Source: CAD feature listing. Evaluate the final solid. Frame: model axes, mm. A direction names the side the tool comes from. Give positions to 0.01 mm unless a question says otherwise; leave off trailing zeros. Loops run counter-clockwise (first coordinate to the right, second up) from the corner with the lowest first, then second, coordinate; pieces in that order, holes last. Notation, with made-up numbers: (35.25, -24.5) -> (73.25, -24.5) arc R21 ccw to (73.25, -19.5) -> close; hole circle Ø7 at (-19.75, -4.75). An arc over 180 degrees is marked (long way). Return JSON: item names as keys, results as strings. Group by question number.
(1) Pin query (flat end, axial travel): pin 1 (5 mm diameter, centred on y = -482.5, z = 15.5, fed in from +X); pin 2 (1 mm diameter, centred on y = -469.5, z = 15.5, fed in from -X); pin 3 (8 mm diameter, centred on x = -2.5, z = 4, fed in from -Y); pin 4 (10 mm diameter, centred on x = -100.5, z = 16, fed in from -Y). Return the tip coordinate at first contact, or that it passes through.
(2) Cut plane B-B on y = -56.5. Return loops of the section in (x, z), then the cut area to 3 significant figures.
(3) Ray query, line 1 (Y direction, x = -10, z = 11); line 2 (X direction, y = -374.5, z = 24.25). Return the intervals inside material, ascending. Write a range as from..to.
(4) Cut plane A-A on x = -73. Return loops of the section in (y, z).
(5) Access query for faces 5 (the face through (-101.6, 661, 13)), 6 (the face through (-153, 317.5, 13)), 7 (the face through (127, -660, 13)). Directions: +Z, -Z, +X, -X, +Y, -Y. A direction counts if a zero-diameter tool reaches every point of the face in a straight line with its end or side. Return the directions, or none.
(6) Draft query along X for faces 1 (the face through (-152, -12.7, 13)), 2 (the face through (127, -455, 13)), 3 (the face through (-127, 455, 13)), 4 (the face through (1, -317.5, 13)). Return one class per face: released by +X, released by -X, zero draft, split by the parting line, or undercut.
(7) Cut plane C-C on z = 16.5. Give the number of separate pieces and of enclosed holes in the cut face, then the cut area to 3 significant figures.
Autodesk Inventor part; units mm, degrees
ref_plane "YZ Plane" through (0, 0, 0) normal (1, 0, 0) x (0, 1, 0)
ref_plane "XZ Plane" through (0, 0, 0) normal (0, 1, 0) x (-1, 0, 0)
ref_plane "XY Plane" through (0, 0, 0) normal (0, 0, 1) x (1, 0, 0)
sketch "Sketch1" plane through (0, 0, 0) normal (0, 0, 1) x (1, 0, 0)
  line L0 (-127, 698.5) -> (-101.6, 698.5)
  line L1 (-101.6, 698.5) -> (-101.6, -698.5)
  line L2 (-101.6, -698.5) -> (-127, -698.5)
  line L3 (-127, -698.5) -> (-127, 698.5)
  line L4 (101.6, 698.5) -> (127, 698.5)
  line L5 (127, 698.5) -> (127, -698.5)
  line L6 (127, -698.5) -> (101.6, -698.5)
  line L7 (101.6, -698.5) -> (101.6, 698.5)
  line L8 (0, 0) -> (0, 143.5331) construction
  line L9 (0, 0) -> (-211.7363, 0) construction
  dimension "d0" = 25.4
  dimension "d1" = 1397
  dimension "d2" = 203.2
extrude "Extrusion1" add sketch "Sketch1" along normal blind 25.4
sketch "Sketch2" plane through (0, 0, 25.4) normal (0, 0, 1) x (1, 0, 0)
  line L0 (-177.8, 622.3) -> (177.8, 622.3)
  line L1 (177.8, 622.3) -> (177.8, 596.9)
  line L2 (177.8, 596.9) -> (-177.8, 596.9)
  line L3 (-177.8, 596.9) -> (-177.8, 622.3)
  line L4 (0, 0) -> (0, 410.334) construction
  line L5 (127, 698.5) -> (101.6, 698.5) construction
  dimension "d5" = 25.4
  dimension "d6" = 355.6
  dimension "d7" = 76.2
extrude "Extrusion2" add sketch "Sketch2" against normal blind 25.4
pattern_linear "Rectangular Pattern1" count 5 spacing 304.8 along (0, -1, 0) of "Extrusion2"
properties part number "Rail zone"
Answers:
{
 "1": {"pin 1": "x = 127", "pin 2": "x = -127", "pin 3": "y = -622.3", "pin 4": "y = -698.5"},
 "2": {"outline": "(-127, 0) -> (-101.6, 0) -> (-101.6, 25.4) -> (-127, 25.4) -> close; (101.6, 0) -> (127, 0) -> (127, 25.4) -> (101.6, 25.4) -> close", "area": "1,290 mm²"},
 "3": {"line 1": "-622.3..-596.9, -317.5..-292.1, -12.7..12.7, 292.1..317.5, 596.9..622.3", "line 2": "-127..-101.6, 101.6..127"},
 "4": {"outline": "(-622.3, 0) -> (-596.9, 0) -> (-596.9, 25.4) -> (-622.3, 25.4) -> close; (-317.5, 0) -> (-292.1, 0) -> (-292.1, 25.4) -> (-317.5, 25.4) -> close; (-12.7, 0) -> (12.7, 0) -> (12.7, 25.4) -> (-12.7, 25.4) -> close; (292.1, 0) -> (317.5, 0) -> (317.5, 25.4) -> (292.1, 25.4) -> close; (596.9, 0) -> (622.3, 0) -> (622.3, 25.4) -> (596.9, 25.4) -> close"},
 "5": {"face 5": "+Z, -Z, +Y", "face 6": "+Z, -Z, -X", "face 7": "+Z, -Z, +X, -Y"},
 "6": {"face 1": "zero draft", "face 2": "released by +X", "face 3": "released by -X", "face 4": "undercut"},
 "7": {"separate pieces": "1", "enclosed holes": "4", "area": "110,000 mm²"}
}
